CAD build for the part. Positions are in the model's coordinates, mm. Face numbers are marked on the shaded views. Round coordinates to 2 decimals unless told otherwise and drop trailing zeros. Write each loop counter-clockwise with the first axis right and the second up, starting at its lowest first coordinate (ties: lowest second). Pieces come first, ordered by that corner, then holes. Notation, with made-up numbers: (11.25, -27) - (70.25, -27) arc R19 cw to (70.25, 4) - close; hole circle Ø9 at (79.25, 20.5). An arc over 180 degrees is marked (long way). Answer in a Markdown table with one row per item.
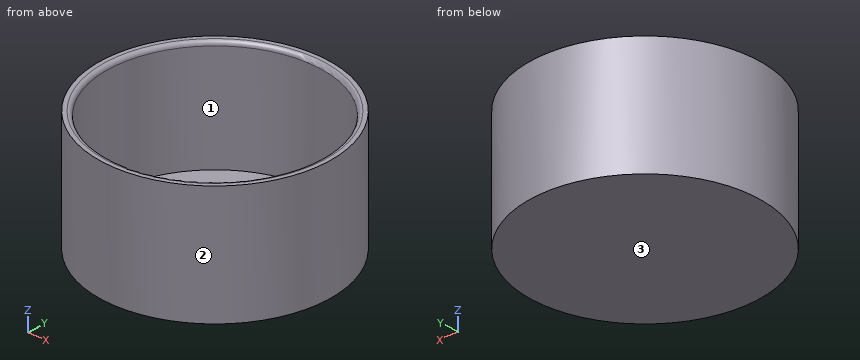
```python
from build123d import *

# Parameters (mm, degrees)
F0_R     = 14.25
F1_DEPTH = 14.7
F2_T     = -1
F3_R     = 0.5


with BuildPart() as f1:
    # F0 (on Top) → F1 (new body)
    with BuildSketch(Plane.XY):
        Circle(F0_R)
    extrude(amount=F1_DEPTH)

    # F2
    f2_openings = [f1.faces().sort_by_distance(p)[0] for p in [
        (0, 0, 14.7),
    ]]
    offset(amount=F2_T, openings=f2_openings)

    # F3
    f3_edges = [f1.edges().sort_by_distance(p)[0] for p in [
        (-13.25, 0, 14.7),
    ]]
    fillet(f3_edges, radius=F3_R)


solid = f1.part
```
Q1. Flat gauge pins, fed straight in: pin 1 (10 mm diameter, centred on x = -1.5, y = -5, fed in from +Z); pin 2 (1 mm diameter, centred on x = -11, y = -11, fed in from -Z); pin 3 (12 mm diameter, centred on x = 5.5, y = -6, fed in from +Z); pin 4 (1 mm diameter, centred on y = 4, z = 10.5, fed in from -X). Where does each tip first touch, or does it go through?
Computed:
| item | result |
|---|---|
| pin 1 | stops at z = 1 |
| pin 2 | passes through |
| pin 3 | stops at z = 14.7 |
| pin 4 | stops at x = -13.81 |
Q2. Saw through at C-C on z = 8.5. List the corners of the cut face in (x, y), then the cut area to 3 significant figures.
Computed:
| item | result |
|---|---|
| outline | circle Ø28.5 at (0, 0); hole circle Ø26.5 at (0, 0) |
| area | 86.4 mm2 |
Q3. Pull direction X, two halves, no side cores. Call the marked faces 1, 2 and 3: released by +X, released by -X, zero draft, split by the parting line, or undercut.
Computed:
| item | result |
|---|---|
| face 1 | undercut |
| face 2 | split by the parting line |
| face 3 | zero draft |
Q4. Saw through at A-A on y = 0. List the corners of the cut face in (x, z).
Computed:
| item | result |
|---|---|
| outline | (-14.25, 0) - (14.25, 0) - (14.25, 14.7) - (13.75, 14.7) arc R0.5 ccw to (13.25, 14.2) - (13.25, 1) - (-13.25, 1) - (-13.25, 14.2) arc R0.5 ccw to (-13.75, 14.7) - (-14.25, 14.7) - close |
Q5. Drill centre lines: line 1 (Y direction, x = 0, z = 5.5); line 2 (Y direction, x = 10, z = 8.5); line 3 (X direction, y = -5, z = 4.25). Where is each one in solid material? Low to high.
Computed:
| item | result |
|---|---|
| line 1 | y = -14.25 to -13.25, 13.25 to 14.25 |
| line 2 | y = -10.15 to -8.69, 8.69 to 10.15 |
| line 3 | x = -13.34 to -12.27, 12.27 to 13.34 |
